Design review of the part built by this model. Coordinates are the model's own, in mm. A direction names the side the tool comes from. Coordinates: 2 decimals unless noted, no trailing zeros. Loops run counter-clockwise (first coordinate to the right, second up) from the corner with the lowest first, then second, coordinate; pieces in that order, holes last. Notation, with made-up numbers: M 38.5,-10.75 L 82.5,-10.75 A13 ccw 82.5,3.25 Z; hole C 28.5,82 d3. An arc over 180 degrees is marked long. Answer as CSV lines item,"result". Start each with the question number.
from build123d import *

# Parameters (mm, degrees)
F1_W    = 0.7335389405
F1_H    = 1.5485889072
F1_H_2  = 1.3186813187
F3_SIZE = 0.33


with BuildPart() as f2:
    # F1 (on Right) → F2 (revolve)
    with BuildSketch(Plane.YZ):
        with BuildLine():
            Line((3.5, 10), (3.5, 11))
            Line((3.5, 11), (0, 11))
            Line((0, 11), (0, 9.1895215866))
            ThreePointArc((0, 9.1895215866), (0.9328753707, 8.9086258319), (1.5555555556, 8.1593406593))
            Line((1.5555555556, 8.1593406593), (2.5, 8.1593406593))
            Line((2.5, 8.1593406593), (2.5, 9.7079295665))
            Line((2.5, 9.7079295665), (2.5, 10))
            Line((2.5, 10), (3.2335389405, 10))
            Line((3.2335389405, 10), (3.5, 10))
        make_face()
        with BuildLine():
            Line((2.5, 5.2920704335), (2.5, 6.8406593407))
            Line((2.5, 6.8406593407), (1.5555555556, 6.8406593407))
            ThreePointArc((1.5555555556, 6.8406593407), (0.9328753707, 6.0913741681), (0, 5.8104784134))
            Line((0, 5.8104784134), (0, 4))
            Line((0, 4), (3.5, 4))
            Line((3.5, 4), (3.5, 5))
            Line((3.5, 5), (3.2335389405, 5))
            Line((3.2335389405, 5), (2.5, 5))
            Line((2.5, 5), (2.5, 5.2920704335))
        make_face()
        with BuildLine():
            Line((-1.5555555556, 6.8406593407), (-2.5, 6.8406593407))
            Line((-2.5, 6.8406593407), (-2.5, 5.2920704335))
            Line((-2.5, 5.2920704335), (-2.5, 5))
            Line((-2.5, 5), (-3.2335389405, 5))
            Line((-3.2335389405, 5), (-3.5, 5))
            Line((-3.5, 5), (-3.5, 4))
            Line((-3.5, 4), (0, 4))
            Line((0, 4), (0, 5.8104784134))
            ThreePointArc((0, 5.8104784134), (-0.9328753707, 6.0913741681), (-1.5555555556, 6.8406593407))
        make_face()
        with BuildLine():
            Line((0, 9.1895215866), (0, 11))
            Line((0, 11), (-3.5, 11))
            Line((-3.5, 11), (-3.5, 10))
            Line((-3.5, 10), (-3.2335389405, 10))
            Line((-3.2335389405, 10), (-2.5, 10))
            Line((-2.5, 10), (-2.5, 9.7079295665))
            Line((-2.5, 9.7079295665), (-2.5, 8.1593406593))
            Line((-2.5, 8.1593406593), (-1.5555555556, 8.1593406593))
            ThreePointArc((-1.5555555556, 8.1593406593), (-0.9328753707, 8.9086258319), (0, 9.1895215866))
        make_face()
        with Locations((2.8667694703, 8.9336351129)):
            Rectangle(F1_W, F1_H)
        with Locations((2.8667694703, 7.5)):
            Rectangle(F1_W, F1_H_2)
        with Locations((2.8667694703, 6.0663648871)):
            Rectangle(F1_W, F1_H)
        with Locations((-2.8667694703, 8.9336351129)):
            Rectangle(F1_W, F1_H)
        with Locations((-2.8667694703, 6.0663648871)):
            Rectangle(F1_W, F1_H)
        with Locations((-2.8667694703, 7.5)):
            Rectangle(F1_W, F1_H_2)
    revolve(axis=Axis((0, 0, 0), (0, -1, 0)))

    # F3
    f3_edges = [f2.edges().sort_by_distance(p)[0] for p in [
        (0, -3.5, -4),
        (0, 3.5, -4),
        (0, 0, 4),
        (0, 3.5, -11),
        (0, -3.5, -11),
        (0, 0, 11),
    ]]
    chamfer(f3_edges, length=F3_SIZE)


with BuildPart() as f2_1:
    # F4: moved
    add(f2.part)


solid = f2_1.part
Item 1: For line 1 along Z through (x, y) = (0, 2.3); line 2 along Y through (x, z) = (-0.5, 7.5), list the stretches that pass through material, from the lowest coordinate up. Write a range as from..to.
Item 2: Mouldability with a two-part tool opening along X and no side actions: class faces 1 (the face through (3.905, 0.044, -0.867)), 2 (the face through (10.74, -0.04, -2.38)), 3 (the face through (-4.5, -3.5, 0)) as released by +X, released by -X, zero draft, split by the parting line, or undercut.
Item 3: Add section A-A (y = -2). Give the boundary of the cut face in (x, z).
Item 4: For faces 4 (the face through (4.695, 2.872, 2.442)), 5 (the face through (3, 3.5, 10)), 6 (the face through (4.695, -2.862, 2.442)), 7 (the face through (-2.451, -2.021, 7.783)), list the 3-axis set-ups (+Z, -Z, +X, -X, +Y, -Y) from which the entire face can be reached by the end or side of a thin tool; tool diameter is ignored.
Item 5: For pin 1 (1.5 mm diameter, centred on y = -0.5, z = -2.5, fed in from -X); pin 2 (2 mm diameter, centred on x = -7, y = -2, fed in from -Z); pin 3 (3 mm diameter, centred on x = -1, z = 8, fed in from +Y); pin 4 (10 mm diameter, centred on x = 0, z = 4, fed in from +Y), all flat-tipped, find the tip position at first contact; note any pin that passes through.
Item 6: Add section B-B (z = 3). Give the number of separate pieces and of enclosed holes in the cut face, plus the area to 3 significant figures.
Response:
1,line 1,"-11..-8.16, -6.84..-4, 4..6.84, 8.16..11"
1,line 2,"-3.23..-2.5, 2.5..3.23"
2,face 1,"undercut"
2,face 2,"split by the parting line"
2,face 3,"zero draft"
3,outline,"C 0,0 d22; C 0,0 d13.68; hole C 0,0 d16.32; hole C 0,0 d8"
4,face 4,"+Y"
4,face 5,"+Z, -Z, +X, -X, +Y"
4,face 6,"-Y"
4,face 7,"none"
5,pin 1,"x = -10.86"
5,pin 2,"z = -9.22"
5,pin 3,"y = 3.23"
5,pin 4,"y = 3.5"
6,separate pieces,"2"
6,enclosed holes,"2"
6,area,"78.1 mm²"
